Can you work these out from the model? Positions are in its coordinate system, mm. Face numbers are marked on the shaded views. A direction names the side the tool comes from. Round coordinates to 2 decimals unless told otherwise and drop trailing zeros. Write each loop counter-clockwise with the first axis right and the second up, starting at its lowest first coordinate (ties: lowest second). Pieces come first, ordered by that corner, then holes.
Q1. If we section it at B-B (x = -25.4): Please give me the cut outline in (y, z) (3 decimals), plus the area to 3 significant figures.
Q2. If we section it at A-A (z = 31.75): Please give me the cut outline in (x, y) (3 decimals).
Q3. For the marked faces 1 and 2, which set-ups out of +Z, -Z, +X, -X, +Y, -Y let a thin tool reach every point of the face, with its end or its side?
Q4. I'm going to push flat-ended pins straight in: pin 1 Ø3 at (y, z) = (3.5, -29) entering from +X; pin 2 Ø8 at (x, y) = (-42, -5.5) entering from +Z (3 decimals); pin 3 Ø5 at (y, z) = (-3.5, 7) entering from -X (3 decimals); pin 4 Ø17 at (x, y) = (-25.4, -31.115) entering from -Z. Where does each tip first touch, or does it pass through?
Q5. If we section it at D-D (x = -13.5): Please give me the cut outline in (y, z) (3 decimals), plus the area to 3 significant figures.
Q6. Please list where these lines run through material, in increasing order: line 1 along Y through (x, z) = (-25.4, -61.5) (3 decimals); line 2 along Z through (x, y) = (-12, -43) (3 decimals); line 3 along X through (y, z) = (2, -22.5) (3 decimals).
Q7. If we section it at C-C (y = -38.1): Give the number of separate pieces and of enclosed holes in the cut face, plus the area to 3 significant figures.
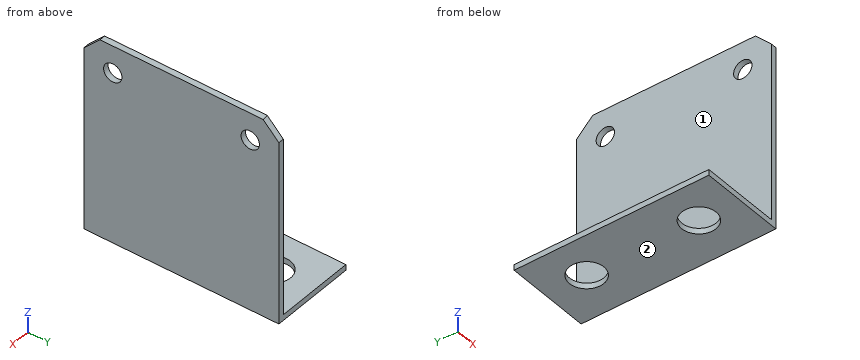
from build123d import *

# Parameters (mm, degrees)
F1_DEPTH  = 3.175
F2_W      = 44.45
F2_H      = 3.175
F3_DEPTH  = 107.95
F4_R      = 5.08
F5_DEPTH  = 3.175
F6_R      = 9.525
F7_DEPTH  = 3.175
F8_DEPTH  = 3.175
F12_DEPTH = 3.175
F12_TAPER = -3


with BuildPart() as f1:
    # F0 (on Right) → F1 (new body)
    with BuildSketch(Plane.YZ):
        Polygon((53.975, 38.1), (28.575, 63.5), (-28.575, 63.5), (-53.975, 38.1), (-53.975, -63.5), (53.975, -63.5), align=None)
    extrude(amount=F1_DEPTH)

    # F2 (on face) → F3 (join, through all)
    with BuildSketch(Plane.XZ.offset(53.975)):
        with Locations((25.4, -61.9125)):
            Rectangle(F2_W, F2_H)
    extrude(amount=-F3_DEPTH)

    # F4 (on face) → F5 (cut, through all)
    with BuildSketch(Plane.YZ.offset(3.175)):
        with Locations((-38.1, 31.75)):
            Circle(F4_R)
        with Locations((38.1, 31.75)):
            Circle(F4_R)
    extrude(amount=-F5_DEPTH, mode=Mode.SUBTRACT)

    # F6 (on face) → F7 (cut, through all)
    with BuildSketch(Plane.XY.offset(-60.325)):
        with Locations((25.4, 31.115)):
            Circle(F6_R)
        with Locations((25.4, -31.115)):
            Circle(F6_R)
    extrude(amount=-F7_DEPTH, mode=Mode.SUBTRACT)

    # F6 (on face) → F8 (cut, through all)
    with BuildSketch(Plane.XY.offset(-60.325)):
        with Locations((25.4, 31.115)):
            Circle(F6_R)
        with Locations((25.4, -31.115)):
            Circle(F6_R)
    extrude(amount=-F8_DEPTH, mode=Mode.SUBTRACT)


with BuildPart() as f9_1:
    # F9: instance of F1
    add(f1.part.mirror(Plane.YZ))

    # F11 (on face) → F12 (cut, through all)
    with BuildSketch(Plane(origin=(-3.175, 0, 0), x_dir=(0, -1, 0), z_dir=(-1, 0, 0))):
        Polygon((28.575, 63.5), (-28.575, 63.5), (-45.085, 46.99), (45.085, 46.99), align=None)
    extrude(amount=-F12_DEPTH, taper=F12_TAPER, mode=Mode.SUBTRACT)


solid = f9_1.part
A:
1. outline: (-53.975, -63.5) - (-40.64, -63.5) - (-40.64, -60.325) - (-53.975, -60.325) - close; (-21.59, -63.5) - (21.59, -63.5) - (21.59, -60.325) - (-21.59, -60.325) - close; (40.64, -63.5) - (53.975, -63.5) - (53.975, -60.325) - (40.64, -60.325) - close
1. area: 222 mm2
2. outline: (-3.175, -53.975) - (0, -53.975) - (0, -43.18) - (-3.175, -43.18) - close; (-3.175, -33.02) - (0, -33.02) - (0, 33.02) - (-3.175, 33.02) - close; (-3.175, 43.18) - (0, 43.18) - (0, 53.975) - (-3.175, 53.975) - close
3. face 1: +Z, -X, +Y, -Y
3. face 2: -Z, +X, -X, +Y, -Y
4. pin 1: stops at x = 0
4. pin 2: stops at z = -60.325
4. pin 3: stops at x = -3.175
4. pin 4: passes through
5. outline: (-53.975, -63.5) - (53.975, -63.5) - (53.975, -60.325) - (-53.975, -60.325) - close
5. area: 343 mm2
6. line 1: y = -53.975 to -40.64, -21.59 to 21.59, 40.64 to 53.975
6. line 2: z = -63.5 to -60.325
6. line 3: x = -3.175 to 0
7. separate pieces: 3
7. enclosed holes: 0
7. area: 418 mm2
